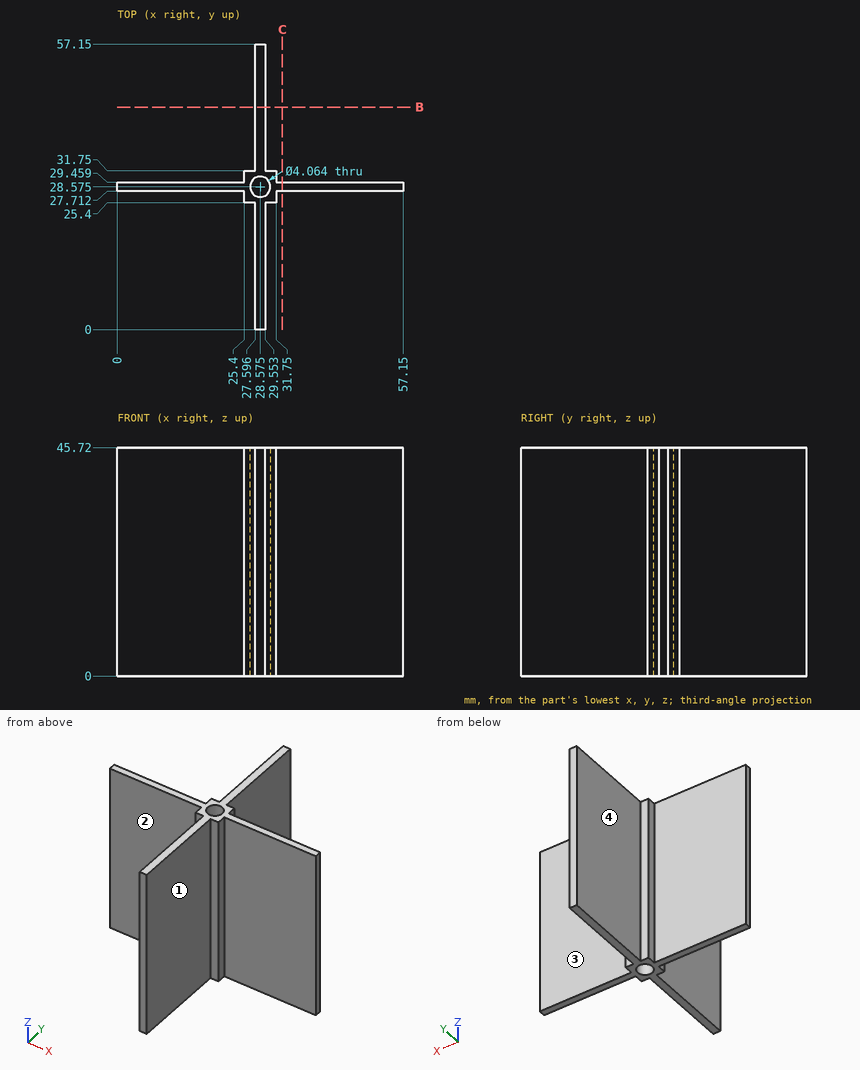
Drawing for the job (mm, zero at the part's lowest x, y, z). A direction names the side the tool comes from. Coordinates: 2 decimals unless noted, no trailing zeros. Order: outer loops, then holes, each group sorted by start corner. A loop starts at its lowest first (then second) coordinate and runs counter-clockwise, first axis right, second up. Notation, with made-up numbers: (46, -2.5) -> (69, -2.5) arc R22 ccw to (69, 21.5) -> close; hole circle Ø7 at (-19, 45). An arc over 180 degrees is marked (long way). One line per item, written item: value.
(1) Tool access for the marked faces 1, 2, 3 and 4: list every direction of +Z, -Z, +X, -X, +Y, -Y with a clear straight run to the whole face (end or side of a thin tool).
Checked values:
face 1: +Z, -Z, +X, -Y
face 2: +Z, -Z, -X, -Y
face 3: +Z, -Z, +X, +Y
face 4: +Z, -Z, -X, +Y
(2) Probe line 1 (Y direction, x = 53.5, z = 11); line 2 (X direction, y = 22, z = 22) (1 decimal); line 3 (X direction, y = 26, z = 43). List the from-to ranges inside material, lowest first. Write a range as [from, to].
Checked values:
line 1: [27.71, 29.46]
line 2: [27.6, 29.6]
line 3: [25.4, 31.75]
(3) Slice it at C-C, the plane x = 33. List the corners of the cut face in (y, z).
Checked values:
outline: (27.71, 0) -> (29.46, 0) -> (29.46, 45.72) -> (27.71, 45.72) -> close
(4) Drop flat-ended pins along their axis: pin 1 Ø20.5 at (y, z) = (9, 13) entering from +X; pin 2 Ø7.5 at (x, z) = (18, 29.5) entering from +Y; pin 3 Ø0.7 at (x, z) = (30.5, 26) entering from +Y. Give the stop position or say it passes through.
Checked values:
pin 1: x = 29.55
pin 2: y = 29.46
pin 3: y = 31.75
(5) Slice it at B-B, the plane y = 44.5. List the corners of the cut face in (x, z) (1 decimal).
Checked values:
outline: (27.6, 0) -> (29.6, 0) -> (29.6, 45.7) -> (27.6, 45.7) -> close
